Print and shaded views of the part. All mm, measured from the part's lowest x, y and z. Give positions to 0.01 mm unless a question says otherwise; leave off trailing zeros. Order: outer loops, then holes, each group sorted by start corner. A loop starts at its lowest first (then second) coordinate and runs counter-clockwise, first axis right, second up. Notation, with made-up numbers: (84.25, 33.5) -> (98.25, 33.5) arc R5 ccw to (98.25, 41.5) -> close; hole circle Ø7 at (73.5, 10.25). An arc over 180 degrees is marked (long way). One line per question, with ' | ' between items. Start each with the question number.
(1) Cut at C-C (z = 3.4). Give the cut face in (x, y) (1 decimal).
(2) Cut at D-D (y = 146.5). Give the cut face in (x, z) (1 decimal).
(3) Pin check, flat tip, straight feed: pin 1 Ø2 at (x, z) = (140, 1.5) entering from +Y. Stop position of the tip, or through.
(4) Drill centre lines: L1, parallel to X at y = 31.5, z = 0.85 (1 decimal); L2, parallel to X at y = 109, z = 0.95 (1 decimal); L3, parallel to Y at x = 100.5, z = 2.7 (1 decimal). Where is each one in solid material? Low to high. Write a range as from..to.
(5) Cut at B-B (x = 70.5). Give the cut face in (y, z) (1 decimal).
(6) Cut at A-A (y = 74). Give the cut face in (x, z), then the cut area to 3 significant figures.
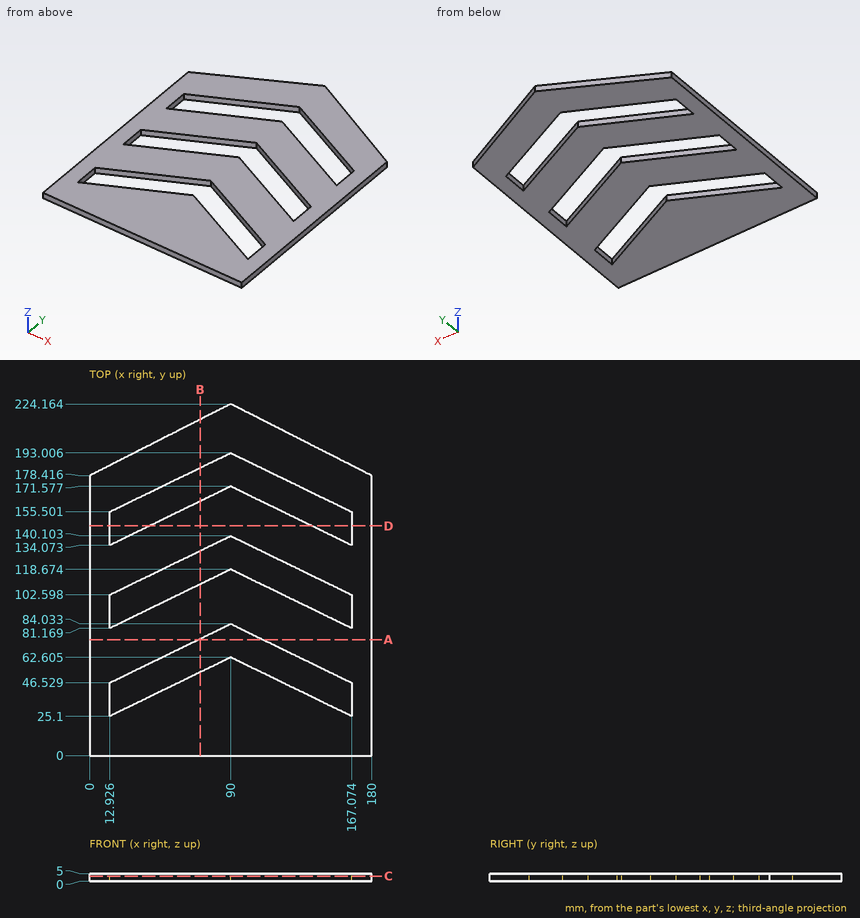
Result set:
1) outline: (0, 0) -> (180, 0) -> (180, 178.4) -> (90, 224.2) -> (0, 178.4) -> close; hole (12.9, 25.1) -> (90, 62.6) -> (167.1, 25.1) -> (167.1, 46.5) -> (90, 84) -> (12.9, 46.5) -> close; hole (12.9, 81.2) -> (90, 118.7) -> (167.1, 81.2) -> (167.1, 102.6) -> (90, 140.1) -> (12.9, 102.6) -> close; hole (12.9, 134.1) -> (90, 171.6) -> (167.1, 134.1) -> (167.1, 155.5) -> (90, 193) -> (12.9, 155.5) -> close
2) outline: (0, 0) -> (12.9, 0) -> (12.9, 5) -> (0, 5) -> close; (38.5, 0) -> (141.5, 0) -> (141.5, 5) -> (38.5, 5) -> close; (167.1, 0) -> (180, 0) -> (180, 5) -> (167.1, 5) -> close
3) pin 1: stops at y = 199.26
4) L1: x = 0..12.9, 26.1..153.9, 167.1..180 | L2: x = 0..26.1, 70.1..109.9, 153.9..180 | L3: y = 0..57.5, 78.9..113.6, 135..166.5, 187.9..218.8
5) outline: (0, 0) -> (53.1, 0) -> (53.1, 5) -> (0, 5) -> close; (74.5, 0) -> (109.2, 0) -> (109.2, 5) -> (74.5, 5) -> close; (130.6, 0) -> (162.1, 0) -> (162.1, 5) -> (130.6, 5) -> close; (183.5, 0) -> (214.3, 0) -> (214.3, 5) -> (183.5, 5) -> close
6) outline: (0, 0) -> (69.38, 0) -> (69.38, 5) -> (0, 5) -> close; (110.62, 0) -> (180, 0) -> (180, 5) -> (110.62, 5) -> close | area: 694 mm2
